Geometry check sheet. Reference: the model listing, model coordinates, mm. A direction names the side the tool comes from. Give positions to 0.01 mm unless a question says otherwise; leave off trailing zeros. Order: outer loops, then holes, each group sorted by start corner. A loop starts at its lowest first (then second) coordinate and runs counter-clockwise, first axis right, second up. Notation, with made-up numbers: M -25,23.25 L 17,23.25 A18 ccw 17,39.25 Z; hole C 12,-30 d2. An arc over 180 degrees is marked long. Put each result on its own line as item: value. Start each with the question number.
Q1. Mould release check, pull along Y, two halves, no side actions. Record for faces 5 (the cylindrical face through (4.44, 8.13, -6.54)), 6 (the flat face through (9, 3, 0)), 7 (the cylindrical face through (4.437, 4.569, 9.386)): +Y half, -Y half, draft (parallel to the pull), parting line (faces both ways), or undercut.
Q2. Go/stop test with flat-tipped pins: pin 1 (1.4 mm diameter, centred on x = 3.5, y = 0.5, fed in from +Z); pin 2 (4 mm diameter, centred on x = 1.5, z = 6.5, fed in from +Y); pin 3 (5 mm diameter, centred on x = 0, y = -6, fed in from -Z). Record where each tip stops, or that it passes through.
Q3. Access from +Z, -Z, +X, -X, +Y, -Y to the whole of each face (thin tool, end or side, straight path). Record for faces 1 (the cylindrical face through (4.437, -4.486, -9.391)), 2 (the cylindrical face through (4.44, -9.02, 5.26)), 3 (the cylindrical face through (4.437, 1.584, -10.286)), 4 (the cylindrical face through (4.437, 9.701, -3.855)).
Q4. Material ranges on L1, parallel to Y at x = 3.75, z = 0; L2, parallel to Z at x = 1.75, y = -1; L3, parallel to Z at x = 7, y = -6.25, recorded low to high.
Q5. Section check A-A on x = -2. Record the cut outline in (y, z), then the cut area to 3 significant figures.
```python
from build123d import *

# Parameters (mm, degrees)
BASPROSKE_W         = 9
BASPROSKE_H         = 11.5
TOOTHCUT_DEPTH      = 19.587630295
TEETHCUTS_COUNT     = 21
TEETHCUTS_ANGLE     = 342.857142857
BORSKE_R            = 2.5
BORE_DEPTH          = 50.0000508
SKETCH1_R           = 7.5
SKETCH1_R_2         = 2.5
BOSS_EXTRUDE1_DEPTH = 4
BOSS_EXTRUDE2_DEPTH = 13


with BuildPart() as part:
    # BasProSke → Base-Revolve (revolve)
    with BuildSketch(Plane(origin=(0, 0, 0), x_dir=(1, 0, 0), z_dir=(0, 1, 0)), mode=Mode.PRIVATE) as base_revolve_sk:
        with Locations((4.5, 5.75)):
            Rectangle(BASPROSKE_W, BASPROSKE_H)
    revolve(base_revolve_sk.sketch.rotate(Axis((-10, 0, 0), (1, 0, 0)), 180), axis=Axis((-10, 0, 0), (1, 0, 0)))

    # TooCutSke → ToothCut (cut, through all)
    with BuildSketch(Plane(origin=(0, 0, 0), x_dir=(0, 0, -1), z_dir=(1, 0, 0))):
        with BuildLine():
            ThreePointArc((0.49526894, 9.235730057), (0, 9.249), (-0.49526894, 9.235730057))
            ThreePointArc((-0.49526894, 9.235730057), (-0.823521057, 10.404716786), (-1.472455249, 11.430954496))
            ThreePointArc((-1.472455249, 11.430954496), (0, 11.5254), (1.472455249, 11.430954496))
            ThreePointArc((1.472455249, 11.430954496), (0.823521057, 10.404716786), (0.49526894, 9.235730057))
        make_face()
    toothcut = extrude(amount=TOOTHCUT_DEPTH, mode=Mode.SUBTRACT)

    # TeethCuts: ToothCut ×21 about axis
    teethcuts_axis = Axis((-10, 0, 0), (1, 0, 0))
    for i in range(1, TEETHCUTS_COUNT):
        add(toothcut.rotate(teethcuts_axis, i * TEETHCUTS_ANGLE / (TEETHCUTS_COUNT - 1)), mode=Mode.SUBTRACT)

    # BorSke → Bore (cut, symmetric)
    with BuildSketch(Plane(origin=(0, 0, 0), x_dir=(0, 0, -1), z_dir=(1, 0, 0))):
        with Locations(Location((0, 0, 0), (0, 0, 180))):
            Circle(BORSKE_R)
    extrude(amount=BORE_DEPTH, both=True, mode=Mode.SUBTRACT)

    # Sketch1 → Boss-Extrude1 (add)
    with BuildSketch(Plane.ZY):
        with Locations(Location((0, 0, 0), (0, 0, 180))):
            Circle(SKETCH1_R)
        Circle(SKETCH1_R_2, mode=Mode.SUBTRACT)
    extrude(amount=BOSS_EXTRUDE1_DEPTH)

    # Sketch2 → Boss-Extrude2 (add, through all)
    with BuildSketch(Plane.ZY.offset(4)):
        with BuildLine():
            Line((-2.1, -1.356465997), (-2.1, 1.356465997))
            ThreePointArc((-2.1, 1.356465997), (-2.5, 0), (-2.1, -1.356465997))
        make_face()
    extrude(amount=-BOSS_EXTRUDE2_DEPTH)


solid = part.part
```
Results found:
1. face 5: +Y half
1. face 6: draft
1. face 7: undercut
2. pin 1: stops at z = 10.81
2. pin 2: stops at y = 10.47
2. pin 3: stops at z = -10.8
3. face 1: +X, -X
3. face 2: +X, -X, -Y
3. face 3: -Z, +X, -X
3. face 4: +X, -X, +Y
4. L1: y = -11.5 to -2.5, 2.5 to 9.25
4. L2: z = -11.46 to -2.1, 2.29 to 11.46
4. L3: z = -8.82 to 8.82
5. outline: C 0,0 d15; hole M -1.36,-2.1 L 1.36,-2.1 A2.5 ccw long Z
5. area: 158 mm^2
